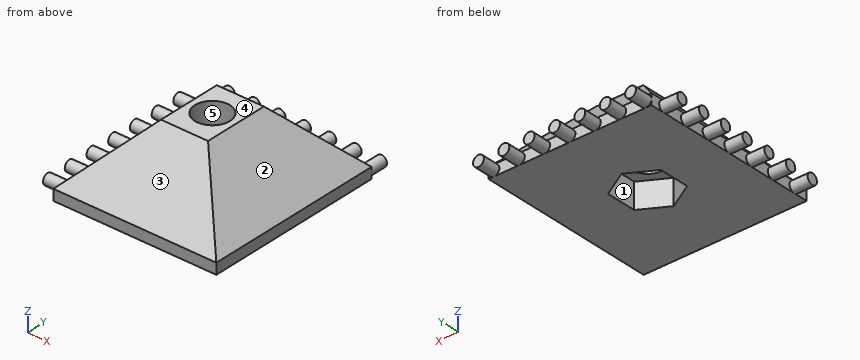
from build123d import *

# Parameters (mm, degrees)
SKETCH_W        = 45
SKETCH_H        = 50
PAD_DEPTH       = 25
CHAMFER_SIZE    = 22
SKETCH001_R     = 4.85
POCKET_DEPTH    = 25.001
SKETCH002_W     = 32.700705
SKETCH002_H     = 10
POCKET001_DEPTH = 45.001
SKETCH003_R     = 1.5
SKETCH003_R_2   = 1.518583
SKETCH003_R_3   = 1.500476
PAD001_DEPTH    = 5
SKETCH004_R     = 1.5
SKETCH004_R_2   = 1.504062
SKETCH004_R_3   = 1.509717
SKETCH004_R_4   = 1.483533
SKETCH004_R_5   = 1.504121
PAD002_DEPTH    = 5
POCKET002_DEPTH = 7


with BuildPart() as part:
    # Sketch → Pad (new body)
    with BuildSketch(Plane.XY):
        Rectangle(SKETCH_W, SKETCH_H)
    extrude(amount=PAD_DEPTH)

    # Chamfer
    chamfer_edges = [part.edges().sort_by_distance(p)[0] for p in [
        (0, 25, 25),
        (-22.5, 0, 25),
        (0, -25, 25),
        (22.5, 0, 25),
    ]]
    chamfer(chamfer_edges, length=CHAMFER_SIZE)

    # Sketch001 → Pocket (cut, through all)
    with BuildSketch(Plane(origin=(0, 0, 0), x_dir=(1, 0, 0), z_dir=(0, 0, -1))):
        Circle(SKETCH001_R)
    extrude(amount=-POCKET_DEPTH, mode=Mode.SUBTRACT)

    # Sketch002 → Pocket001 (cut, through all)
    with BuildSketch(Plane(origin=(-22.5, 0, 0), x_dir=(0, -1, 0), z_dir=(-1, 0, 0))):
        with Locations((-0.350352, 24)):
            Rectangle(SKETCH002_W, SKETCH002_H)
    extrude(amount=-POCKET001_DEPTH, mode=Mode.SUBTRACT)

    # Sketch003 → Pad001 (new body)
    with BuildSketch(Plane(origin=(0, 25, 0), x_dir=(-1, 0, 0), z_dir=(0, 1, 0))):
        with Locations((-21, 1.5)):
            Circle(SKETCH003_R)
        with Locations((-14, 1.5)):
            Circle(SKETCH003_R_2)
        with Locations((0, 1.5)):
            Circle(SKETCH003_R)
        with Locations((-7, 1.5)):
            Circle(SKETCH003_R)
        with Locations((7, 1.5)):
            Circle(SKETCH003_R_3)
        with Locations((14, 1.5)):
            Circle(SKETCH003_R)
        with Locations((21, 1.5)):
            Circle(SKETCH003_R)
    extrude(amount=PAD001_DEPTH)

    # Sketch004 → Pad002 (new body)
    with BuildSketch(Plane(origin=(-22.5, 0, 0), x_dir=(0, -1, 0), z_dir=(-1, 0, 0))):
        with Locations((0, 1.5)):
            Circle(SKETCH004_R)
        with Locations((-7, 1.5)):
            Circle(SKETCH004_R_2)
        with Locations((-14, 1.5)):
            Circle(SKETCH004_R)
        with Locations((-21, 1.5)):
            Circle(SKETCH004_R_3)
        with Locations((7, 1.5)):
            Circle(SKETCH004_R_4)
        with Locations((14, 1.5)):
            Circle(SKETCH004_R)
        with Locations((21, 1.5)):
            Circle(SKETCH004_R_5)
    extrude(amount=PAD002_DEPTH)

    # Sketch005 → Pocket002 (cut)
    with BuildSketch(Plane(origin=(0, 0, 0), x_dir=(1, 0, 0), z_dir=(0, 0, -1))):
        Polygon((7.3, -4.214657), (7.3, 4.214657), (0, 8.429314), (-7.3, 4.214657), (-7.3, -4.214657), (0, -8.429314), align=None)
    extrude(amount=-POCKET002_DEPTH, mode=Mode.SUBTRACT)


solid = part.part
Could you check a few things on this model? Use its own coordinates, in mm. Face numbers are marked on the shaded views. A direction names the side the tool comes from. Give positions to 0.01 mm unless a question says otherwise; leave off trailing zeros. Order: outer loops, then holes, each group sorted by start corner. A loop starts at its lowest first (then second) coordinate and runs counter-clockwise, first axis right, second up. Notation, with made-up numbers: (49.25, 79) - (88.25, 79) arc R26 ccw to (88.25, 109) - close; hole circle Ø3 at (63.5, -15.75). An arc over 180 degrees is marked (long way). One line per item, written item: value. Start each with the question number.
1. Imagine slicing it at D-D on z = 11. List the corners of the cut face in (x, y) for me.
2. Thinking about a two-plate mould opening in Y: for the marked faces 3, 4 and 5, which applies, +Y half, -Y half, draft (parallel to the pull), parting line (faces both ways), or undercut?
3. Imagine slicing it at C-C on x = -11.5. List the corners of the cut face in (y, z) for me, plus the area to 3 significant figures.
4. If I drill on probe 1 along X at (y, z) = (0, 13); probe 2 along Z at (x, y) = (-2, -21); probe 3 along X at (y, z) = (0, 15.5), over which ranges is the centre line in solid material (lowest first)?
5. For P1, Ø1.5, axis at y = 23.5, z = 2, coming from the -X side; P2, Ø1.5, axis at x = -4, y = -10.5, coming from the -Z side; P3, Ø8, axis at x = 15, z = 10.5, coming from the -Y side, each with a flat end and sliding along its axis, tell me the tip position at first contact or that it passes through.
6. For the marked faces 1 and 2, which set-ups out of +Z, -Z, +X, -X, +Y, -Y let a thin tool reach every point of the face, with its end or its side?
7. Imagine slicing it at B-B on y = -3. List the corners of the cut face in (x, z) for me.
8. Imagine slicing it at A-A on z = 6.25. List the corners of the cut face in (x, y) for me.
Values:
1. outline: (-14.5, -17) - (14.5, -17) - (14.5, 17) - (-14.5, 17) - close; hole circle Ø9.7 at (0, 0)
2. face 3: -Y half
2. face 4: draft
2. face 5: undercut
3. outline: (-25, 0) - (25, 0) - (25, 3) - (14, 14) - (-14, 14) - (-25, 3) - close
3. area: 579 mm²
4. probe 1: -12.5 to -4.85, 4.85 to 12.5
4. probe 2: 0 to 7
4. probe 3: -10 to -4.85, 4.85 to 10
5. P1: x = -22.5
5. P2: z = 0
5. P3: y = -21.5
6. face 1: -Z
6. face 2: +Z, +X, +Y, -Y
7. outline: (-22.5, 0) - (-7.3, 0) - (-7.3, 7) - (-3.81, 7) - (-3.81, 19) - (-6.5, 19) - (-22.5, 3) - close; (3.81, 7) - (7.3, 7) - (7.3, 0) - (22.5, 0) - (22.5, 3) - (6.5, 19) - (3.81, 19) - close
8. outline: (-19.25, -21.75) - (19.25, -21.75) - (19.25, 21.75) - (-19.25, 21.75) - close; hole (-7.3, -4.21) - (0, -8.43) - (7.3, -4.21) - (7.3, 4.21) - (0, 8.43) - (-7.3, 4.21) - close
